```python
from build123d import *

# Parameters (mm, degrees)
F1_DEPTH = 2
F0_R     = 3
F0_R_2   = 1.5
F2_DEPTH = 5
F4_DEPTH = 5
F5_DEPTH = 8
F6_DEPTH = 4
F7_DEPTH = 15
F8_DEPTH = 15
F3_W     = 1
F3_H     = 6
F9_DEPTH = 5


with BuildPart() as f1:
    # F0 (on Top) → F1 (new body)
    with BuildSketch(Plane.XY):
        with BuildLine():
            Line((-14, -20), (-2.69212803, -20))
            ThreePointArc((-2.69212803, -20), (0, -18.323800087), (2.69212803, -20))
            Line((2.69212803, -20), (14, -20))
            ThreePointArc((14, -20), (14.7071067812, -19.7071067812), (15, -19))
            Line((15, -19), (15, -15.5))
            ThreePointArc((15, -15.5), (14.4142135624, -16.9142135624), (13, -17.5))
            Line((13, -17.5), (-13, -17.5))
            ThreePointArc((-13, -17.5), (-14.4142135624, -16.9142135624), (-15, -15.5))
            Line((-15, -15.5), (-15, -19))
            ThreePointArc((-15, -19), (-14.7071067812, -19.7071067812), (-14, -20))
        make_face()
    extrude(amount=F1_DEPTH)

    # F0 (on Top) → F2 (join)
    with BuildSketch(Plane.XY):
        with BuildLine():
            Line((2.7598104581, -22.5), (16.5, -22.5))
            ThreePointArc((16.5, -22.5), (17.9142135624, -21.9142135624), (18.5, -20.5))
            Line((18.5, -20.5), (18.5, 3.5))
            ThreePointArc((18.5, 3.5), (18.2071067812, 4.2071067812), (17.5, 4.5))
            ThreePointArc((17.5, 4.5), (16.7928932188, 4.7928932188), (16.5, 5.5))
            Line((16.5, 5.5), (16.5, 17.5694916397))
            Line((16.5, 17.5694916397), (16.5, 20.5))
            ThreePointArc((16.5, 20.5), (15.9142135624, 21.9142135624), (14.5, 22.5))
            Line((14.5, 22.5), (-16.5, 22.5))
            ThreePointArc((-16.5, 22.5), (-17.9142135624, 21.9142135624), (-18.5, 20.5))
            Line((-18.5, 20.5), (-18.5, 17.5694916397))
            Line((-18.5, 17.5694916397), (-18.5, -20.5))
            ThreePointArc((-18.5, -20.5), (-17.9142135624, -21.9142135624), (-16.5, -22.5))
            Line((-16.5, -22.5), (-2.7598104581, -22.5))
            ThreePointArc((-2.7598104581, -22.5), (-2.9989011853, -21.2426109214), (-2.69212803, -20))
            Line((-2.69212803, -20), (-14, -20))
            ThreePointArc((-14, -20), (-14.7071067812, -19.7071067812), (-15, -19))
            Line((-15, -19), (-15, -15.5))
            Line((-15, -15.5), (-15, 2.5))
            ThreePointArc((-15, 2.5), (-14.4142135624, 3.9142135624), (-13, 4.5))
            Line((-13, 4.5), (-12, 4.5))
            ThreePointArc((-12, 4.5), (-10.5857864376, 5.0857864376), (-10, 6.5))
            Line((-10, 6.5), (-10, 8.1054256072))
            ThreePointArc((-10, 8.1054256072), (-9.6405519552, 9.2493614806), (-8.6914107177, 9.9821118409))
            Line((-8.6914107177, 9.9821118409), (6.3085892823, 15.5084276303))
            ThreePointArc((6.3085892823, 15.5084276303), (8.1439358734, 15.2722933519), (9, 13.6317413967))
            Line((9, 13.6317413967), (9, 2.5))
            ThreePointArc((9, 2.5), (9.2928932188, 1.7928932188), (10, 1.5))
            Line((10, 1.5), (14, 1.5))
            ThreePointArc((14, 1.5), (14.7071067812, 1.2071067812), (15, 0.5))
            Line((15, 0.5), (15, -15.5))
            Line((15, -15.5), (15, -19))
            ThreePointArc((15, -19), (14.7071067812, -19.7071067812), (14, -20))
            Line((14, -20), (2.69212803, -20))
            ThreePointArc((2.69212803, -20), (2.9220184881, -20.6442355536), (3, -21.323800087))
            ThreePointArc((3, -21.323800087), (2.9393393283, -21.9240369676), (2.7598104581, -22.5))
        make_face()
        with BuildLine():
            ThreePointArc((-12.5, 17.5694916397), (-15.5, 14.5694916397), (-18.5, 17.5694916397))
            ThreePointArc((-18.5, 17.5694916397), (-15.5, 20.5694916397), (-12.5, 17.5694916397))
        make_face(mode=Mode.SUBTRACT)
        with Locations((13.5, 17.5694916397)):
            Circle(F0_R, mode=Mode.SUBTRACT)
        with BuildLine():
            ThreePointArc((2.69212803, -20), (0, -18.323800087), (-2.69212803, -20))
            Line((-2.69212803, -20), (-0.7053746024, -20))
            ThreePointArc((-0.7053746024, -20), (0, -19.823800087), (0.7053746024, -20))
            Line((0.7053746024, -20), (2.69212803, -20))
        make_face()
        with BuildLine():
            ThreePointArc((-2.69212803, -20), (-2.9989011853, -21.2426109214), (-2.7598104581, -22.5))
            Line((-2.7598104581, -22.5), (-0.9308886961, -22.5))
            ThreePointArc((-0.9308886961, -22.5), (-1.4939342005, -21.1890388), (-0.7053746024, -20))
            Line((-0.7053746024, -20), (-2.69212803, -20))
        make_face()
        with BuildLine():
            Line((0.9308886961, -22.5), (2.7598104581, -22.5))
            ThreePointArc((2.7598104581, -22.5), (2.9393393283, -21.9240369676), (3, -21.323800087))
            ThreePointArc((3, -21.323800087), (2.9220184881, -20.6442355536), (2.69212803, -20))
            Line((2.69212803, -20), (0.7053746024, -20))
            ThreePointArc((0.7053746024, -20), (1.2860913466, -20.5518097708), (1.5, -21.323800087))
            ThreePointArc((1.5, -21.323800087), (1.3502468375, -21.9771250275), (0.9308886961, -22.5))
        make_face()
        with BuildLine():
            ThreePointArc((-2.7598104581, -22.5), (0, -24.323800087), (2.7598104581, -22.5))
            Line((2.7598104581, -22.5), (0.9308886961, -22.5))
            ThreePointArc((0.9308886961, -22.5), (0, -22.823800087), (-0.9308886961, -22.5))
            Line((-0.9308886961, -22.5), (-2.7598104581, -22.5))
        make_face()
        with BuildLine():
            ThreePointArc((-12.5, 17.5694916397), (-15.5, 20.5694916397), (-18.5, 17.5694916397))
            ThreePointArc((-18.5, 17.5694916397), (-15.5, 14.5694916397), (-12.5, 17.5694916397))
        make_face()
        with Locations((-15.5, 17.5694916397)):
            Circle(F0_R_2, mode=Mode.SUBTRACT)
        with Locations((13.5, 17.5694916397)):
            Circle(F0_R)
        with Locations((13.5, 17.5694916397)):
            Circle(F0_R_2, mode=Mode.SUBTRACT)
    extrude(amount=F2_DEPTH)

    # F3 (on face) → F4 (join)
    with BuildSketch(Plane.XY.offset(5)):
        with BuildLine():
            ThreePointArc((-18.5, -14.5), (-18.2071067812, -15.2071067812), (-17.5, -15.5))
            Line((-17.5, -15.5), (-16, -15.5))
            ThreePointArc((-16, -15.5), (-15.2928932188, -15.2071067812), (-15, -14.5))
            Line((-15, -14.5), (-15, 2.5))
            ThreePointArc((-15, 2.5), (-14.4142135624, 3.9142135624), (-13, 4.5))
            Line((-13, 4.5), (-12, 4.5))
            ThreePointArc((-12, 4.5), (-10.5857864376, 5.0857864376), (-10, 6.5))
            Line((-10, 6.5), (-10, 8.1054256072))
            ThreePointArc((-10, 8.1054256072), (-9.6405519552, 9.2493614806), (-8.6914107177, 9.9821118409))
            Line((-8.6914107177, 9.9821118409), (-11.5, 8.9473684211))
            Line((-11.5, 8.9473684211), (-11.5, 8.5))
            ThreePointArc((-11.5, 8.5), (-11.7928932188, 7.7928932188), (-12.5, 7.5))
            Line((-12.5, 7.5), (-16.5, 7.5))
            ThreePointArc((-16.5, 7.5), (-17.9142135624, 6.9142135624), (-18.5, 5.5))
            Line((-18.5, 5.5), (-18.5, -14.5))
        make_face()
    extrude(amount=F4_DEPTH)

    # F3 (on face) → F5 (join)
    with BuildSketch(Plane.XY.offset(5)):
        with BuildLine():
            Line((4.5, 22.5), (-9.5, 22.5))
            ThreePointArc((-9.5, 22.5), (-10.9142135624, 21.9142135624), (-11.5, 20.5))
            Line((-11.5, 20.5), (-11.5, 8.9473684211))
            Line((-11.5, 8.9473684211), (-8.6914107177, 9.9821118409))
            Line((-8.6914107177, 9.9821118409), (6.3085892823, 15.5084276303))
            Line((6.3085892823, 15.5084276303), (6.5, 15.5789473684))
            Line((6.5, 15.5789473684), (6.5, 20.5))
            ThreePointArc((6.5, 20.5), (5.9142135624, 21.9142135624), (4.5, 22.5))
        make_face()
    extrude(amount=F5_DEPTH)

    # F3 (on face) → F6 (join)
    with BuildSketch(Plane.XY.offset(5)):
        with BuildLine():
            ThreePointArc((10, -19.5), (9.5, -19.6339745962), (9.1339745962, -20))
            Line((9.1339745962, -20), (14, -20))
            ThreePointArc((14, -20), (14.5, -19.8660254038), (14.8660254038, -19.5))
            Line((14.8660254038, -19.5), (10, -19.5))
        make_face()
        with BuildLine():
            ThreePointArc((9, -21.5), (9.2928932188, -22.2071067812), (10, -22.5))
            Line((10, -22.5), (16.5, -22.5))
            ThreePointArc((16.5, -22.5), (17.9142135624, -21.9142135624), (18.5, -20.5))
            ThreePointArc((18.5, -20.5), (18.2071067812, -19.7928932188), (17.5, -19.5))
            Line((17.5, -19.5), (14.8660254038, -19.5))
            ThreePointArc((14.8660254038, -19.5), (14.5, -19.8660254038), (14, -20))
            Line((14, -20), (9.1339745962, -20))
            ThreePointArc((9.1339745962, -20), (9.0340741737, -20.2411809549), (9, -20.5))
            Line((9, -20.5), (9, -21.5))
        make_face()
    extrude(amount=-F6_DEPTH)

    # F3 (on face) → F7 (join)
    with BuildSketch(Plane.XY.offset(5)):
        with BuildLine():
            ThreePointArc((10, -19.5), (9.5, -19.6339745962), (9.1339745962, -20))
            Line((9.1339745962, -20), (14, -20))
            ThreePointArc((14, -20), (14.5, -19.8660254038), (14.8660254038, -19.5))
            Line((14.8660254038, -19.5), (10, -19.5))
        make_face()
        with BuildLine():
            ThreePointArc((9, -21.5), (9.2928932188, -22.2071067812), (10, -22.5))
            Line((10, -22.5), (16.5, -22.5))
            ThreePointArc((16.5, -22.5), (17.9142135624, -21.9142135624), (18.5, -20.5))
            ThreePointArc((18.5, -20.5), (18.2071067812, -19.7928932188), (17.5, -19.5))
            Line((17.5, -19.5), (14.8660254038, -19.5))
            ThreePointArc((14.8660254038, -19.5), (14.5, -19.8660254038), (14, -20))
            Line((14, -20), (9.1339745962, -20))
            ThreePointArc((9.1339745962, -20), (9.0340741737, -20.2411809549), (9, -20.5))
            Line((9, -20.5), (9, -21.5))
        make_face()
    extrude(amount=F7_DEPTH)

    # F3 (on face) → F8 (join)
    with BuildSketch(Plane.XY.offset(5)):
        with BuildLine():
            ThreePointArc((17.5, 1.5), (18.2071067812, 1.7928932188), (18.5, 2.5))
            Line((18.5, 2.5), (18.5, 3.5))
            ThreePointArc((18.5, 3.5), (18.2071067812, 4.2071067812), (17.5, 4.5))
            Line((17.5, 4.5), (13.25, 4.5))
            Line((13.25, 4.5), (12.25, 4.5))
            Line((12.25, 4.5), (10, 4.5))
            ThreePointArc((10, 4.5), (9.2928932188, 4.2071067812), (9, 3.5))
            Line((9, 3.5), (9, 2.5))
            ThreePointArc((9, 2.5), (9.2928932188, 1.7928932188), (10, 1.5))
            Line((10, 1.5), (12.25, 1.5))
            Line((12.25, 1.5), (13.25, 1.5))
            Line((13.25, 1.5), (14, 1.5))
            Line((14, 1.5), (17.5, 1.5))
        make_face()
        with BuildLine():
            ThreePointArc((15.5, 10.5), (16.2071067812, 10.7928932188), (16.5, 11.5))
            ThreePointArc((16.5, 11.5), (16.2071067812, 12.2071067812), (15.5, 12.5))
            Line((15.5, 12.5), (10, 12.5))
            ThreePointArc((10, 12.5), (9.2928932188, 12.2071067812), (9, 11.5))
            ThreePointArc((9, 11.5), (9.2928932188, 10.7928932188), (10, 10.5))
            Line((10, 10.5), (12.25, 10.5))
            Line((12.25, 10.5), (13.25, 10.5))
            Line((13.25, 10.5), (15.5, 10.5))
        make_face()
    extrude(amount=F8_DEPTH)

    # F3 (on face) → F9 (join)
    with BuildSketch(Plane.XY.offset(5)):
        with Locations((12.75, 7.5)):
            Rectangle(F3_W, F3_H)
    extrude(amount=F9_DEPTH)


solid = f1.part
```
Can you work these out from the model? Positions are in its coordinate system, mm. A direction names the side the tool comes from. Give positions to 0.01 mm unless a question says otherwise; leave off trailing zeros. Loops run counter-clockwise (first coordinate to the right, second up) from the corner with the lowest first, then second, coordinate; pieces in that order, holes last. Notation, with made-up numbers: M 16.5,-19.75 L 73.5,-19.75 A9 cw 73.5,-15.75 Z; hole C 77.5,-9 d11. An arc over 180 degrees is marked long. Answer in a Markdown table with one row per item.
1. For pin 1 Ø3.5 at (x, y) = (4, -17.5) entering from +Z; pin 2 Ø8 at (x, y) = (-2.5, -20) entering from +Z; pin 3 Ø0.5 at (x, y) = (12.5, 9) entering from +Z; pin 4 Ø12 at (y, z) = (9, 13.5) entering from -X, each with a flat end and sliding along its axis, tell me the tip position at first contact or that it passes through.
Taken from the geometry:
| item | result |
|---|---|
| pin 1 | stops at z = 2 |
| pin 2 | stops at z = 5 |
| pin 3 | stops at z = 10 |
| pin 4 | stops at x = -18.5 |
2. If I drill on line 1 along Y through (x, z) = (13.5, 3.75); line 2 along Y through (x, z) = (-15.5, 2.35); line 3 along Y through (x, z) = (11, 9), over which ranges is the centre line in solid material (lowest first)?
Taken from the geometry:
| item | result |
|---|---|
| line 1 | y = -22.5 to -19.5, 1.5 to 16.07, 19.07 to 22.5 |
| line 2 | y = -22.5 to 16.07, 19.07 to 22.5 |
| line 3 | y = -22.5 to -19.5, 1.5 to 4.5, 10.5 to 12.5 |
3. Suppose I cut it at A-A on y = -7. Write out the boundary of the cut face in (x, z).
Taken from the geometry:
| item | result |
|---|---|
| outline | M -18.5,0 L -15,0 L -15,10 L -18.5,10 Z; M 15,0 L 18.5,0 L 18.5,5 L 15,5 Z |
4. Suppose I cut it at B-B on z = 15. Write out the boundary of the cut face in (x, y), plus the area to 3 significant figures.
Taken from the geometry:
| item | result |
|---|---|
| outline | M 9,-21.5 A1 ccw 10,-22.5 L 16.5,-22.5 A2 ccw 18.5,-20.5 A1 ccw 17.5,-19.5 L 10,-19.5 A1 ccw 9,-20.5 Z; M 9,2.5 A1 ccw 10,1.5 L 17.5,1.5 A1 ccw 18.5,2.5 L 18.5,3.5 A1 ccw 17.5,4.5 L 10,4.5 A1 ccw 9,3.5 Z; M 10,10.5 L 15.5,10.5 A1 ccw 15.5,12.5 L 10,12.5 A1 ccw Z |
| area | 68.8 mm² |
5. Suppose I cut it at D-D on z = 4.25. Count the separate pieces of the cut face and the enclosed holes in it, plus the area to 3 significant figures.
Taken from the geometry:
| item | result |
|---|---|
| separate pieces | 1 |
| enclosed holes | 4 |
| area | 745 mm² |
6. Which directions (+Z, -Z, +X, -X, +Y, -Y) give clear straight access to the entire face, cutting with the end or side of a thin tool? Please do faces 4 (the flat face through (-14, 7.5, 7)), 5 (the flat face through (15, 7, 5)), 6 (the flat face through (14, 1.5, 10)), 7 (the flat face through (-12.5, 4.5, 4.9)), 8 (the flat face through (9, -21, 12)).
Taken from the geometry:
| item | result |
|---|---|
| face 4 | +Z, -X, +Y |
| face 5 | +Z, +X |
| face 6 | +Z |
| face 7 | +Z, -Z |
| face 8 | +Z, -X, +Y, -Y |
7. Thinking about a two-plate mould opening in Y: for faces 1 (the flat face through (-6, -21, 5)), 2 (the cylindrical face through (-17.9, 21.93, 2.46)), 3 (the cylindrical face through (0.047, -18.324, 3.479)), which applies, released by +Y, released by -Y, zero draft, split by the parting line, or undercut?
Taken from the geometry:
| item | result |
|---|---|
| face 1 | zero draft |
| face 2 | released by +Y |
| face 3 | undercut |
8. Suppose I cut it at C-C on x = -5.5. Write out the boundary of the cut face in (y, z), plus the area to 3 significant figures.
Taken from the geometry:
| item | result |
|---|---|
| outline | M -22.5,0 L -17.5,0 L -17.5,2 L -20,2 L -20,5 L -22.5,5 Z; M 11.16,0 L 22.5,0 L 22.5,13 L 11.16,13 Z |
| area | 165 mm² |
